```python
from build123d import *

# Parameters (mm, degrees)
F4_DEPTH = 26.001
F3_W     = 16
F3_H     = 2.2
F5_DEPTH = 23


with BuildPart() as f1:
    # F0 (on Front) → F1 (revolve)
    with BuildSketch(Plane.XZ):
        Polygon((-13, 0), (-11.8, 0), (-11.8, 7.1), (-11.8, 9.6), (-11.8, 13.4200323373), (-12.6346228644, 17), (-13, 17), align=None)
        Polygon((-11.8, 9.6), (-11.8, 7.1), (-10.3265667208, 7.1), (-10.9094091813, 9.6), align=None)
    revolve(axis=Axis((0, 0, 8.5), (0, 0, 1)))

    # F3 (on offset) → F4 (cut, through all)
    with BuildSketch(Plane.XZ.offset(13)):
        with BuildLine():
            add(Edge.make_bspline(
                [(-9.9011575398, 17.5226589309), (-10.2594239129, 18.308274348), (-11.2375961727, 20.4532348174), (-2.9366854637, 21.7150870272), (14.527182625, 22.1780936044), (24.3522467857, 14.4704645715), (20.6659768906, 6.8973925089), (20.535883493, 6.3841777406), (18.5511625655, 4.67363665), (17.0875235032, 3.4121924222)],
                knots=[0, 0, 0, 0, 0.0870359311, 0.2376336152, 0.4909532197, 0.6806586372, 0.8308190148, 0.8752369186, 1, 1, 1, 1], degree=3))
            add(Edge.make_bspline(
                [(-9.9011575398, 17.5226589309), (-1.0566617884, 14.9280194281), (5.2971986995, 15.8914451573), (12.9903821447, 8.1766160182), (17.0875235032, 3.4121924222)],
                knots=[0, 0, 0, 0, 0.5060819041, 1, 1, 1, 1], degree=3))
        make_face()
    extrude(amount=-F4_DEPTH, mode=Mode.SUBTRACT)

    # F3 (on offset) → F5 (cut)
    with BuildSketch(Plane.XZ.offset(13)):
        with Locations((0, 8.3)):
            Rectangle(F3_W, F3_H)
    extrude(amount=-F5_DEPTH, mode=Mode.SUBTRACT)


solid = f1.part
```
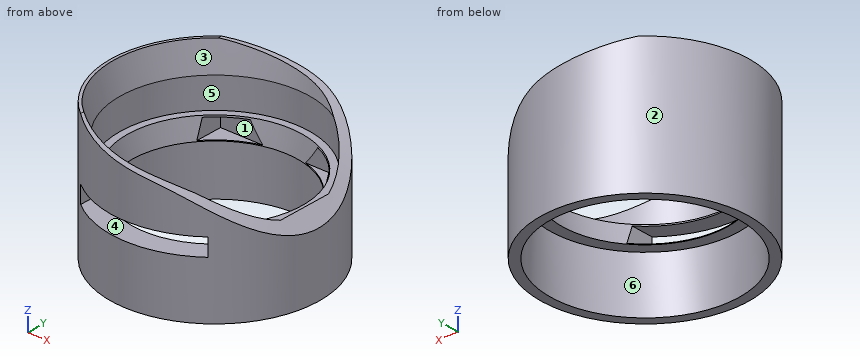
Build history of the part. All positions in model axes, mm. Face numbers are marked on the shaded views. A direction names the side the tool comes from. Coordinates: 2 decimals unless noted, no trailing zeros. Order: outer loops, then holes, each group sorted by start corner. A loop starts at its lowest first (then second) coordinate and runs counter-clockwise, first axis right, second up.
Item 1: Saw through at B-B on x = -1. State how many separate pieces and enclosed holes the cut face has, then the cut area to 3 significant figures.
Filled in:
separate pieces: 3
enclosed holes: 0
area: 36.9 mm2
Item 2: Drop flat-ended pins along their axis: pin 1 Ø5 at (x, z) = (10, 12.5) entering from -Y; pin 2 Ø1 at (x, y) = (4.5, 9) entering from +Z; pin 3 Ø7 at (x, y) = (2, -8.5) entering from +Z (3 decimals). Give the stop position or say it passes through.
Filled in:
pin 1: stops at y = -10.62
pin 2: stops at z = 7.2
pin 3: stops at z = 14.905
Item 3: Drill centre lines: L1, parallel to X at y = 0, z = 4.5; L2, parallel to X at y = 0, z = 11.8. Where is each one in solid material? Low to high.
Filled in:
L1: x = -13 to -11.8, 11.8 to 13
L2: x = -13 to -11.8
Item 4: Mould opens along Y. For the marked faces 1, 2 and 3 say: released by +Y, released by -Y, zero draft, split by the parting line, or undercut.
Filled in:
face 1: released by -Y
face 2: split by the parting line
face 3: undercut
Item 5: Saw through at A-A on z = 2.25. List the corners of the cut face in (x, y), then the cut area to 3 significant figures.
Filled in:
outline: circle Ø26 at (0, 0); hole circle Ø23.6 at (0, 0)
area: 93.5 mm2
Item 6: Tool access for the marked faces 4, 5 and 6: list every direction of +Z, -Z, +X, -X, +Y, -Y with a clear straight run to the whole face (end or side of a thin tool).
Filled in:
face 4: -Y
face 5: +Z
face 6: -Z
